Check sheet for the modelled part. Datum: model origin and axes. Units: mm. A direction names the side the tool comes from. Coordinates: 2 decimals unless noted, no trailing zeros. Loops run counter-clockwise (first coordinate to the right, second up) from the corner with the lowest first, then second, coordinate; pieces in that order, holes last.
```python
from build123d import *

# Parameters (mm, degrees)
EXTRUDE_1_DEPTH = 3
FILLET_1_R      = 1.27


with BuildPart() as part:
    # 스케치1 → 보스-돌출1 (new body)
    with BuildSketch(Plane.XY):
        with BuildLine():
            Line((-1.4475, 5.825839477), (1.4475, 5.825839477))
            Line((1.4475, 5.825839477), (1.4475, 2.825839477))
            ThreePointArc((1.4475, 2.825839477), (2.528752179, 1.919905575), (3.110851973, 0.635))
            ThreePointArc((3.110851973, 0.635), (7.073084861, 0), (3.110851973, -0.635))
            ThreePointArc((3.110851973, -0.635), (2.533845793, -1.913178115), (1.4625, -2.818105525))
            Line((1.4625, -2.818105525), (1.4625, -9.057688378))
            ThreePointArc((1.4625, -9.057688378), (3.012624602, -8.666297826), (4.471273428, -8.011762536))
            ThreePointArc((4.471273428, -8.011762536), (13.073084861, 0), (4.471273428, 8.011762536))
            ThreePointArc((4.471273428, 8.011762536), (0, 9.175), (-4.471273428, 8.011762536))
            ThreePointArc((-4.471273428, 8.011762536), (-13.073084861, 0), (-4.471273428, -8.011762536))
            ThreePointArc((-4.471273428, -8.011762536), (-3.012624602, -8.666297826), (-1.4625, -9.057688378))
            Line((-1.4625, -9.057688378), (-1.4625, -2.818105525))
            ThreePointArc((-1.4625, -2.818105525), (-2.533845793, -1.913178115), (-3.110851973, -0.635))
            ThreePointArc((-3.110851973, -0.635), (-7.073084861, 0), (-3.110851973, 0.635))
            ThreePointArc((-3.110851973, 0.635), (-2.528752179, 1.919905575), (-1.4475, 2.825839477))
            Line((-1.4475, 2.825839477), (-1.4475, 5.825839477))
        make_face()
    extrude(amount=EXTRUDE_1_DEPTH)

    # 필렛1
    fillet_1_edges = [part.edges().sort_by_distance(p)[0] for p in [
        (-3.110851973, 0.635, 1.5),
        (-3.110851973, -0.635, 1.5),
        (-1.4625, -9.057688378, 1.5),
        (1.4625, -9.057688378, 1.5),
        (3.110851973, -0.635, 1.5),
        (3.110851973, 0.635, 1.5),
    ]]
    fillet(fillet_1_edges, radius=FILLET_1_R)


solid = part.part
```
1) Section check B-B on x = -6. Enter the section's corners in (y, z), plus the area to 3 significant figures.
Answer sheet:
outline: (-7.97, 0) - (-1.79, 0) - (-1.79, 3) - (-7.97, 3) - close; (1.79, 0) - (7.97, 0) - (7.97, 3) - (1.79, 3) - close
area: 37.1 mm2
2) Section check A-A on y = 0. Enter the section's corners in (x, z).
Answer sheet:
outline: (-13.07, 0) - (-7.07, 0) - (-7.07, 3) - (-13.07, 3) - close; (7.07, 0) - (13.07, 0) - (13.07, 3) - (7.07, 3) - close
3) Section check C-C on y = 6.5. Enter the section's corners in (x, z), plus the area to 3 significant figures.
Answer sheet:
outline: (-9.76, 0) - (9.76, 0) - (9.76, 3) - (-9.76, 3) - close
area: 58.6 mm2
4) Set-up check for faces 4 (the flat face through (1.448, 4, 1)), 5 (the cylindrical face through (1.97, 2.49, 1.48)), 6 (the cylindrical face through (0.065, 9.175, 1.479)): record each of +Z, -Z, +X, -X, +Y, -Y from which the full face is reachable in a straight line by a thin tool's end or side.
Answer sheet:
face 4: +Z, -Z, -Y
face 5: +Z, -Z
face 6: +Z, -Z, +Y
5) Scan lines: line 1 (Y direction, x = 5, z = 0.5); line 2 (X direction, y = 1.75, z = 0.7); line 3 (X direction, y = 0.75, z = 2.5). Record each from-to range of solid material in increasing order.
Answer sheet:
line 1: y = -8.03 to -2.03, 2.03 to 8.03
line 2: x = -12.88 to -6.07, -4.01 to -2.79, 2.79 to 4.01, 6.07 to 12.88
line 3: x = -13.04 to -6.93, 6.93 to 13.04
6) Depth check by flat-ended pin: pin 1 (5.5 mm diameter, centred on x = -5.04, y = 0, fed in from +Z); pin 2 (0.9 mm diameter, centred on y = 4.5, z = 1.5, fed in from -X); pin 3 (0.9 mm diameter, centred on y = -4.5, z = 2, fed in from +X); pin 4 (1.5 mm diameter, centred on y = -4.5, z = 2, fed in from -X). Enter the tip coordinate at first touch or a pass-through.
Answer sheet:
pin 1: stops at z = 3
pin 2: stops at x = -11.98
pin 3: stops at x = 11.98
pin 4: stops at x = -12.14
7) Mould release check, pull along Y, two halves, no side actions. Record for faces 1 (the cylindrical face through (-3.842, -8.332, 1.479)), 2 (the cylindrical face through (7.072, 0.059, 1.479)), 3 (the flat face through (3, 2, 0)): +Y half, -Y half, draft (parallel to the pull), parting line (faces both ways), or undercut.
Answer sheet:
face 1: -Y half
face 2: undercut
face 3: draft
